Design review of the part shown in the three views and the two pictorial views. Dimensions are in mm from the part's minimum x, y and z. Round coordinates to 2 decimals unless told otherwise and drop trailing zeros. Write each loop counter-clockwise with the first axis right and the second up, starting at its lowest first coordinate (ties: lowest second). Pieces come first, ordered by that corner, then holes. Notation, with made-up numbers: (37.5, -14.5) -> (74.5, -14.5) arc R33 ccw to (74.5, 22.5) -> close; hole circle Ø9 at (46.25, 13). An arc over 180 degrees is marked (long way). One line per question, with ' | ' between items. Start each with the question number.
1) Consider section D-D (x = 30.5). Give the boundary of the cut face in (y, z).
2) Consider section B-B (x = 1.5). Give the boundary of the cut face in (y, z), then the cut area to 3 significant figures.
3) Consider section C-C (z = 1.5). Give the boundary of the cut face in (x, y), then the cut area to 3 significant figures.
4) Consider section A-A (z = 15). Give the boundary of the cut face in (x, y), then the cut area to 3 significant figures.
5) For probe 1 along X at (y, z) = (3.45, 26.5); probe 2 along Y at (x, z) = (15.5, 10.5); probe 3 along X at (y, z) = (1.4, 10), list the stretches that pass through material, from the lowest coordinate up.
6) Insertion check: pin 1 Ø1.2 at (y, z) = (1.5, 13.5) entering from +X; pin 2 Ø2.5 at (x, z) = (1.5, 1.5) entering from -Y. Each pin has a flat end and moves straight along its axis. Give the tip position at first contact, or say it passes through.
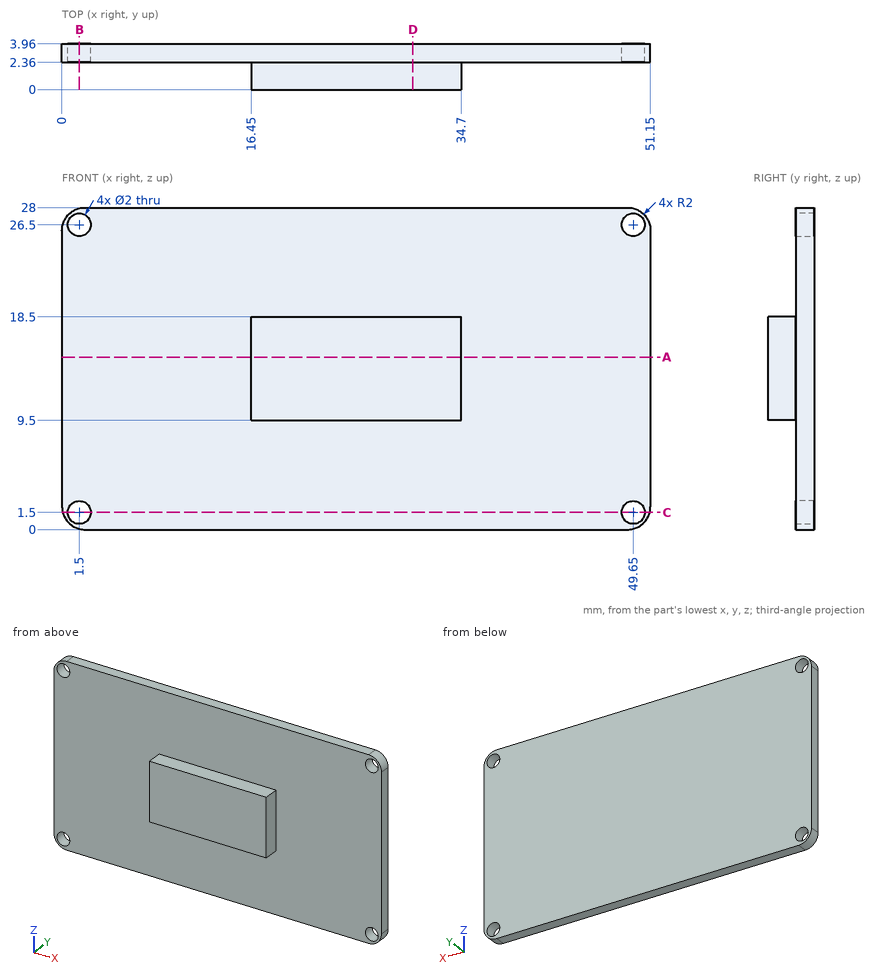
From the geometry:
1) outline: (0, 9.5) -> (2.36, 9.5) -> (2.36, 0) -> (3.96, 0) -> (3.96, 28) -> (2.36, 28) -> (2.36, 18.5) -> (0, 18.5) -> close
2) outline: (2.36, 0.06) -> (3.96, 0.06) -> (3.96, 0.5) -> (2.36, 0.5) -> close; (2.36, 2.5) -> (3.96, 2.5) -> (3.96, 25.5) -> (2.36, 25.5) -> close; (2.36, 27.5) -> (3.96, 27.5) -> (3.96, 27.94) -> (2.36, 27.94) -> close | area: 38.2 mm2
3) outline: (0.06, 2.36) -> (0.5, 2.36) -> (0.5, 3.96) -> (0.06, 3.96) -> close; (2.5, 2.36) -> (48.65, 2.36) -> (48.65, 3.96) -> (2.5, 3.96) -> close; (50.65, 2.36) -> (51.09, 2.36) -> (51.09, 3.96) -> (50.65, 3.96) -> close | area: 75.2 mm2
4) outline: (0, 2.36) -> (16.45, 2.36) -> (16.45, 0) -> (34.7, 0) -> (34.7, 2.36) -> (51.15, 2.36) -> (51.15, 3.96) -> (0, 3.96) -> close | area: 125 mm2
5) probe 1: x = 0.06 to 0.5, 2.5 to 48.65, 50.65 to 51.09 | probe 2: y = 2.36 to 3.96 | probe 3: x = 16.45 to 34.7
6) pin 1: stops at x = 34.7 | pin 2: stops at y = 2.36
